Autodesk Inventor part; units mm, degrees
ref_plane "Start Plane" through (0, 0, 0) normal (1, 0, 0) x (0, 1, 0)
ref_plane "XZ Plane" through (0, 0, 0) normal (0, 1, 0) x (-1, 0, 0)
ref_plane "XY Plane" through (0, 0, 0) normal (0, 0, 1) x (1, 0, 0)
sketch "Main Sketch" plane through (0, 0, 0) normal (0, 0, 1) x (1, 0, 0)
  line L0 (0, 0) -> (80, 0)
  line L1 (0, 0) -> (0, 3)
  line L2 (80, 3) -> (80, 0)
  line L3 (0, 3) -> (80, 3)
  dimension "d3" = 6
revolve "Revolution1" add sketch "Main Sketch" angle 360 about axis through (0, 0, 0) along (1, 0, 0)
chamfer "Chamfer1" distance 0.5 angle 45 1 edges at (0, -3, 0) measured on face at (53.3333, 2.9612, -0.4812)
chamfer "Chamfer2" distance 0.5 angle 45 1 edges at (80, -3, 0) measured on face at (53.5, 2.9903, -0.2414)
properties part number "Shaft" material "Steel"
Verification items for the finished model (mm, model axes). Coordinates: 2 decimals unless noted, no trailing zeros. Loops run counter-clockwise (first coordinate to the right, second up) from the corner with the lowest first, then second, coordinate; pieces in that order, holes last. Notation, with made-up numbers: (-28, 70) -> (-12, 70) arc R6 ccw to (-12, 75) -> close; hole circle Ø4 at (-35, 9.5). An arc over 180 degrees is marked (long way). Write each question's results on one line, items separated by ' | '.
Item 1: Gauge pin test, flat end, axial feed: pin 1 (1.5 mm diameter, centred on x = 58.5, y = 1.5, fed in from -Z). Record the tip position at first contact, or that the pin passes through.
Found:
pin 1: stops at z = -2.9
Item 2: Section check A-A, the plane x = 48. Enter the section's corners in (y, z), plus the area to 3 significant figures.
Found:
outline: circle Ø6 at (0, 0) | area: 28.3 mm2
Item 3: Material ranges on L1, parallel to Y at x = 48, z = -0.1; L2, parallel to Z at x = 39, y = -0.3; L3, parallel to Z at x = 40, y = 1.65, recorded low to high.
Found:
L1: y = -3 to 3 | L2: z = -2.98 to 2.98 | L3: z = -2.51 to 2.51
